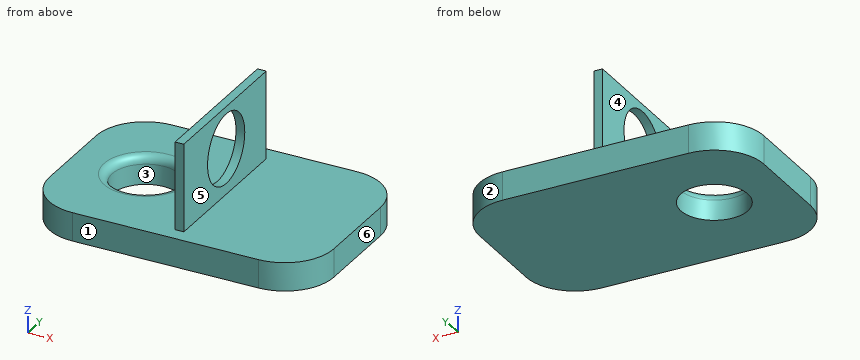
```python
from build123d import *

# Parameters (mm, degrees)
F0_R     = 12.59962
F1_DEPTH = 10.668
F2_R     = 3.066051
F3_W     = 57.973618
F3_H     = 34.38655
F3_R     = 13.105167
F4_DEPTH = 3.302


with BuildPart() as f1:
    # F0 (on Top) → F1 (new body)
    with BuildSketch(Plane.XY):
        with BuildLine():
            Line((34.315242, 34.36793), (-35.594401, 34.36793))
            ThreePointArc((-35.594401, 34.36793), (-48.613899, 28.975077), (-54.006752, 15.955579))
            Line((-54.006752, 15.955579), (-54.006752, -16.882243))
            ThreePointArc((-54.006752, -16.882243), (-48.613897, -29.901747), (-35.594393, -35.294602))
            Line((-35.594393, -35.294602), (34.315242, -35.294602))
            ThreePointArc((34.315242, -35.294602), (47.334745, -29.901747), (52.7276, -16.882243))
            Line((52.7276, -16.882243), (52.7276, 15.955572))
            ThreePointArc((52.7276, 15.955572), (47.334745, 28.975075), (34.315242, 34.36793))
        make_face()
        with Locations((-26.912455, 0)):
            Circle(F0_R, mode=Mode.SUBTRACT)
    extrude(amount=F1_DEPTH)

    # F2
    f2_edges = [f1.edges().sort_by_distance(p)[0] for p in [
        (-39.512074, 0, 10.668),
    ]]
    fillet(f2_edges, radius=F2_R)

    # F3 (on Right) → F4 (join)
    with BuildSketch(Plane.YZ):
        with Locations((-0.793372, 26.436993)):
            Rectangle(F3_W, F3_H)
        with Locations((0, 27.82166)):
            Circle(F3_R, mode=Mode.SUBTRACT)
    extrude(amount=F4_DEPTH)


solid = f1.part
```
Build history of the part. All positions in model axes, mm. Face numbers are marked on the shaded views. A direction names the side the tool comes from. Round coordinates to 2 decimals unless told otherwise and drop trailing zeros. Loops run counter-clockwise (first coordinate to the right, second up) from the corner with the lowest first, then second, coordinate; pieces in that order, holes last.
Item 1: Drill centre lines: line 1 along Z through (x, y) = (2, 0); line 2 along Z through (x, y) = (24, -15); line 3 along Y through (x, z) = (-22, 4.5). Where is each one in solid material? Low to high.
Item 2: Saw through at C-C (z = 37). List the corners of the cut face in (x, y), then the cut area to 3 significant figures.
Item 3: Which spindle directions (+Z, -Z, +X, -X, +Y, -Y) get a long thin tool onto all of the face, cutting with end or side? Do the marked faces 4, 5 and 6. Say none if no direction does.
Item 4: Saw through at D-D (y = 22.5). List the corners of the cut face in (x, z), then the cut area to 3 significant figures.
Item 5: Saw through at A-A (y = 0). List the corners of the cut face in (x, z), then the cut area to 3 significant figures.
Item 6: Pin check, flat tips, straight feed: P1, Ø10, axis at y = -12, z = 29, coming from the +X side; P2, Ø2.5, axis at x = 1.5, z = 23, coming from the -Y side; P3, Ø1, axis at x = -17, y = -11, coming from the +Z side. Stop position of each tip, or through.
Item 7: Saw through at B-B (z = 3). List the corners of the cut face in (x, y).
Item 8: Two-plate mould, pull along Y, no slides. Class the marked faces 1, 2 and 3: released by +Y, released by -Y, zero draft, split by the parting line, or undercut.
Worked answers:
1. line 1: z = 0 to 14.72, 40.93 to 43.63
1. line 2: z = 0 to 10.67
1. line 3: y = -35.29 to -11.6, 11.6 to 34.37
2. outline: (0, -29.78) - (3.3, -29.78) - (3.3, -9.35) - (0, -9.35) - close; (0, 9.35) - (3.3, 9.35) - (3.3, 28.19) - (0, 28.19) - close
2. area: 130 mm2
3. face 4: +Z, -X, +Y, -Y
3. face 5: +Z, +X, +Y, -Y
3. face 6: +Z, -Z, +X, +Y, -Y
4. outline: (-52.8, 0) - (51.53, 0) - (51.53, 10.67) - (3.3, 10.67) - (3.3, 43.63) - (0, 43.63) - (0, 10.67) - (-52.8, 10.67) - close
4. area: 1,220 mm2
5. outline: (-54.01, 0) - (-39.51, 0) - (-39.51, 7.6) arc R3.07 ccw to (-42.58, 10.67) - (-54.01, 10.67) - close; (-14.31, 0) - (52.73, 0) - (52.73, 10.67) - (3.3, 10.67) - (3.3, 14.72) - (0, 14.72) - (0, 10.67) - (-11.25, 10.67) arc R3.07 ccw to (-14.31, 7.6) - close; (0, 40.93) - (3.3, 40.93) - (3.3, 43.63) - (0, 43.63) - close
5. area: 888 mm2
6. P1: stops at x = 3.3
6. P2: stops at y = -29.78
6. P3: stops at z = 10.65
7. outline: (-54.01, -16.88) arc R18.41 ccw to (-35.59, -35.29) - (34.32, -35.29) arc R18.41 ccw to (52.73, -16.88) - (52.73, 15.96) arc R18.41 ccw to (34.32, 34.37) - (-35.59, 34.37) arc R18.41 ccw to (-54.01, 15.96) - close; hole circle Ø25.2 at (-26.91, 0)
8. face 1: released by -Y
8. face 2: released by +Y
8. face 3: undercut
